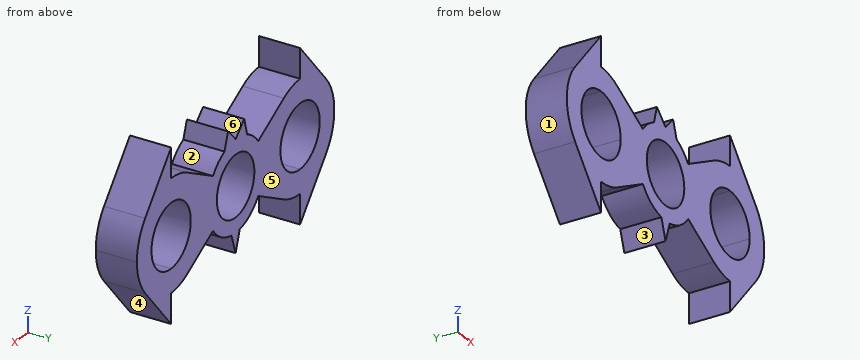
```python
from build123d import *

# Parameters (mm, degrees)
F0_R     = 11.1087126895
F1_DEPTH = 15


with BuildPart() as f1:
    # F0 (on Front) → F1 (new body)
    with BuildSketch(Plane.XZ):
        with BuildLine():
            ThreePointArc((13.4054841173, -9.6794165893), (15.7329987638, -5.0863405143), (16.5347546074, 0))
            ThreePointArc((16.5347546074, 0), (15.7329987638, 5.0863405143), (13.4054841173, 9.6794165893))
            ThreePointArc((13.4054841173, 9.6794165893), (10.3636127764, 12.8838519143), (6.5817506, 15.1683443054))
            ThreePointArc((6.5817506, 15.1683443054), (3.3610458965, 16.1895484931), (0, 16.5347546074))
            Line((0, 16.5347546074), (-6.84138025, 15.0530271442))
            ThreePointArc((-6.84138025, 15.0530271442), (-10.4739105293, 12.7943467263), (-13.4054841173, 9.6794165893))
            ThreePointArc((-13.4054841173, 9.6794165893), (-16.5347546074, 0), (-13.4054841173, -9.6794165893))
            ThreePointArc((-13.4054841173, -9.6794165893), (-8.6057957477, -14.1187247823), (-2.46063304, -16.3506389774))
            ThreePointArc((-2.46063304, -16.3506389774), (-1.2337558027, -16.4886614541), (0, -16.5347546074))
            ThreePointArc((0, -16.5347546074), (1.2337558027, -16.4886614541), (2.46063304, -16.3506389774))
            ThreePointArc((2.46063304, -16.3506389774), (8.6057957477, -14.1187247823), (13.4054841173, -9.6794165893))
        make_face()
        Circle(F0_R, mode=Mode.SUBTRACT)
        with BuildLine():
            ThreePointArc((13.4054841173, 9.6794165893), (15.7329987638, 5.0863405143), (16.5347546074, 0))
            ThreePointArc((16.5347546074, 0), (15.7329987638, -5.0863405143), (13.4054841173, -9.6794165893))
            Line((13.4054841173, -9.6794165893), (28.5778386551, -17.8569645029))
            ThreePointArc((28.5778386551, -17.8569645029), (17.9168171415, 0), (28.5778386551, 17.8569645029))
            Line((28.5778386551, 17.8569645029), (13.4054841173, 9.6794165893))
        make_face()
        with BuildLine():
            ThreePointArc((0, 16.5347546074), (3.3610458965, 16.1895484931), (6.5817506, 15.1683443054))
            Line((6.5817506, 15.1683443054), (4.477564806, 21.3183363497))
            Line((4.477564806, 21.3183363497), (0, 16.5347546074))
        make_face()
        with BuildLine():
            ThreePointArc((38.2023292013, 20.2855120599), (33.2392489705, 19.6690069438), (28.5778386551, 17.8569645029))
            ThreePointArc((28.5778386551, 17.8569645029), (17.9168171415, 0), (28.5778386551, -17.8569645029))
            ThreePointArc((28.5778386551, -17.8569645029), (33.2392489705, -19.6690069438), (38.2023292013, -20.2855120599))
            Line((38.2023292013, -20.2855120599), (38.2023292013, -11.637699008))
            ThreePointArc((38.2023292013, -11.637699008), (26.5646301933, 0), (38.2023292013, 11.637699008))
            Line((38.2023292013, 11.637699008), (38.2023292013, 20.2855120599))
        make_face()
        with BuildLine():
            Line((0, -23.6800604716), (2.46063304, -16.3506389774))
            ThreePointArc((2.46063304, -16.3506389774), (1.2337558027, -16.4886614541), (0, -16.5347546074))
            Line((0, -16.5347546074), (0, -23.6800604716))
        make_face()
        with BuildLine():
            Line((-6.84138025, 15.0530271442), (0, 16.5347546074))
            ThreePointArc((0, 16.5347546074), (-3.5, 16.1600776585), (-6.84138025, 15.0530271442))
        make_face()
        with BuildLine():
            ThreePointArc((-6.84138025, 15.0530271442), (-3.5, 16.1600776585), (0, 16.5347546074))
            Line((0, 16.5347546074), (-5.1105132536, 21.3183363497))
            Line((-5.1105132536, 21.3183363497), (-6.84138025, 15.0530271442))
        make_face()
        with BuildLine():
            Line((38.2023292013, 31.1350713114), (38.2023292013, 20.2855120599))
            ThreePointArc((38.2023292013, 20.2855120599), (46.6697685138, 18.4337861282), (53.5913383502, 13.216671175))
            Line((53.5913383502, 13.216671175), (38.2023292013, 31.1350713114))
        make_face()
        with BuildLine():
            ThreePointArc((53.5913383502, 13.216671175), (46.6697685138, 18.4337861282), (38.2023292013, 20.2855120599))
            Line((38.2023292013, 20.2855120599), (38.2023292013, 11.637699008))
            ThreePointArc((38.2023292013, 11.637699008), (46.4314250873, 8.229095886), (49.8400282094, 0))
            ThreePointArc((49.8400282094, 0), (46.4314250873, -8.229095886), (38.2023292013, -11.637699008))
            Line((38.2023292013, -11.637699008), (38.2023292013, -20.2855120599))
            ThreePointArc((38.2023292013, -20.2855120599), (46.6697685138, -18.4337861282), (53.5913383502, -13.216671175))
            ThreePointArc((53.5913383502, -13.216671175), (57.2243681327, -7.0472714171), (58.4878412612, 0))
            ThreePointArc((58.4878412612, 0), (57.2243681327, 7.0472714171), (53.5913383502, 13.216671175))
        make_face()
        with BuildLine():
            Line((0, -23.6800604716), (0, -16.5347546074))
            ThreePointArc((0, -16.5347546074), (-1.2337558027, -16.4886614541), (-2.46063304, -16.3506389774))
            Line((-2.46063304, -16.3506389774), (0, -23.6800604716))
        make_face()
        with BuildLine():
            ThreePointArc((53.5913383502, -13.216671175), (46.6697685138, -18.4337861282), (38.2023292013, -20.2855120599))
            Line((38.2023292013, -20.2855120599), (38.2023292013, -31.1350713114))
            Line((38.2023292013, -31.1350713114), (53.5913383502, -13.216671175))
        make_face()
        with BuildLine():
            ThreePointArc((-13.4054841173, -9.6794165893), (-16.5347546074, 0), (-13.4054841173, 9.6794165893))
            Line((-13.4054841173, 9.6794165893), (-28.5778386551, 17.8569645029))
            ThreePointArc((-28.5778386551, 17.8569645029), (-20.7848133254, 10.3986605023), (-17.9168171415, 0))
            ThreePointArc((-17.9168171415, 0), (-20.7848133254, -10.3986605023), (-28.5778386551, -17.8569645029))
            Line((-28.5778386551, -17.8569645029), (-13.4054841173, -9.6794165893))
        make_face()
        with BuildLine():
            ThreePointArc((-17.9168171415, 0), (-20.7848133254, 10.3986605023), (-28.5778386551, 17.8569645029))
            ThreePointArc((-28.5778386551, 17.8569645029), (-33.2392489705, 19.6690069438), (-38.2023292013, 20.2855120599))
            Line((-38.2023292013, 20.2855120599), (-38.2023292013, 11.637699008))
            ThreePointArc((-38.2023292013, 11.637699008), (-29.9732333154, 8.229095886), (-26.5646301933, 0))
            ThreePointArc((-26.5646301933, 0), (-29.9732333154, -8.229095886), (-38.2023292013, -11.637699008))
            Line((-38.2023292013, -11.637699008), (-38.2023292013, -20.2855120599))
            ThreePointArc((-38.2023292013, -20.2855120599), (-33.2392489705, -19.6690069438), (-28.5778386551, -17.8569645029))
            ThreePointArc((-28.5778386551, -17.8569645029), (-20.7848133254, -10.3986605023), (-17.9168171415, 0))
        make_face()
        with BuildLine():
            Line((-38.2023292013, 11.637699008), (-38.2023292013, 20.2855120599))
            ThreePointArc((-38.2023292013, 20.2855120599), (-46.6697685138, 18.4337861282), (-53.5913383502, 13.216671175))
            ThreePointArc((-53.5913383502, 13.216671175), (-58.4878412612, 0), (-53.5913383502, -13.216671175))
            ThreePointArc((-53.5913383502, -13.216671175), (-46.6697685138, -18.4337861282), (-38.2023292013, -20.2855120599))
            Line((-38.2023292013, -20.2855120599), (-38.2023292013, -11.637699008))
            ThreePointArc((-38.2023292013, -11.637699008), (-49.8400282094, 0), (-38.2023292013, 11.637699008))
        make_face()
        with BuildLine():
            ThreePointArc((-53.5913383502, 13.216671175), (-46.6697685138, 18.4337861282), (-38.2023292013, 20.2855120599))
            Line((-38.2023292013, 20.2855120599), (-38.2023292013, 31.1350713114))
            Line((-38.2023292013, 31.1350713114), (-53.5913383502, 13.216671175))
        make_face()
        with BuildLine():
            Line((-38.2023292013, -31.1350713114), (-38.2023292013, -20.2855120599))
            ThreePointArc((-38.2023292013, -20.2855120599), (-46.6697685138, -18.4337861282), (-53.5913383502, -13.216671175))
            Line((-53.5913383502, -13.216671175), (-38.2023292013, -31.1350713114))
        make_face()
    extrude(amount=F1_DEPTH)


solid = f1.part
```
Here's how the part is built. I have some questions about the finished solid (model axes, mm). Face numbers are marked on the shaded views. A direction names the side the tool comes from. Coordinates: 2 decimals unless noted, no trailing zeros. Write each loop counter-clockwise with the first axis right and the second up, starting at its lowest first coordinate (ties: lowest second). Pieces come first, ordered by that corner, then holes. Notation, with made-up numbers: (-33, 40) -> (-1, 40) arc R20 ccw to (-1, 60) -> close; hole circle Ø10 at (53, -18.5). An arc over 180 degrees is marked (long way). Use a Markdown table: item, result. Add a question column.
(1) If we section it at B-B, the plane y = -11.5: State how many separate pieces and enclosed holes the cut face has, and give its area (3 significant figures).
(2) If we section it at C-C, the plane x = 36: Write out the boundary of the cut face in (y, z).
(3) If we section it at A-A, the plane x = -46: Write out the boundary of the cut face in (y, z), and give its area (3 significant figures).
(4) If we section it at D-D, the plane x = -19: Write out the boundary of the cut face in (y, z), and give its area (3 significant figures).
(5) I'm going to push flat-ended pins straight in: P1, Ø1.5, axis at x = -20.5, y = -7.5, coming from the +Z side; P2, Ø8.5, axis at y = -4.5, z = 26.5, coming from the +X side; P3, Ø5, axis at x = -32.5, y = -9.5, coming from the +Z side; P4, Ø4, axis at x = -2.5, z = -15, coming from the +Y side. Where does each tip first touch, or does it pass through?
(6) For the marked faces 1, 2 and 3, which set-ups out of +Z, -Z, +X, -X, +Y, -Y let a thin tool reach every point of the face, with its end or its side?
(7) We'd pull the mould along X, two halves only. Please class the marked faces 4, 5 and 6: +X half, -X half, draft (parallel to the pull), parting line (faces both ways), or undercut.
(8) Please list where these lines run through material, in increasing order: line 1 (X direction, y = -3.25, z = -8); line 2 (X direction, y = -8.75, z = -12); line 3 (Z direction, x = 34, y = -6.75).
Outcome:
| question | item | result |
|---|---|---|
| 1 | separate pieces | 1 |
| 1 | enclosed holes | 3 |
| 1 | area | 2,720 mm^2 |
| 2 | outline | (-15, -20.17) -> (0, -20.17) -> (0, -11.43) -> (-15, -11.43) -> close; (-15, 11.43) -> (0, 11.43) -> (0, 20.17) -> (-15, 20.17) -> close |
| 3 | outline | (-15, -22.06) -> (0, -22.06) -> (0, -8.64) -> (-15, -8.64) -> close; (-15, 8.64) -> (0, 8.64) -> (0, 22.06) -> (-15, 22.06) -> close |
| 3 | area | 403 mm^2 |
| 4 | outline | (-15, -12.69) -> (0, -12.69) -> (0, 12.69) -> (-15, 12.69) -> close |
| 4 | area | 381 mm^2 |
| 5 | P1 | stops at z = 13.91 |
| 5 | P2 | stops at x = 45.83 |
| 5 | P3 | stops at z = 20.03 |
| 5 | P4 | stops at y = 0 |
| 6 | face 1 | -X, +Y, -Y |
| 6 | face 2 | +Z, +Y, -Y |
| 6 | face 3 | -Z, +Y, -Y |
| 7 | face 4 | +X half |
| 7 | face 5 | draft |
| 7 | face 6 | undercut |
| 8 | line 1 | x = -56.84 to -46.65, -29.75 to -7.71, 7.71 to 29.75, 46.65 to 56.84 |
| 8 | line 2 | x = -54.56 to -17.71, -11.38 to 11.38, 17.71 to 54.56 |
| 8 | line 3 | z = -19.85 to -10.85, 10.85 to 19.85 |
